```python
from build123d import *

# Parameters (mm, degrees)
SKETCH1_W           = 17.5
SKETCH1_H           = 22.5
BOSS_EXTRUDE1_DEPTH = 1.7
SKETCH2_W           = 6.644971707
SKETCH2_H           = 6.310332844
BOSS_EXTRUDE2_DEPTH = 2.75
SKETCH3_W           = 4.852263512
SKETCH3_H           = 6.382041172
BOSS_EXTRUDE3_DEPTH = 2


with BuildPart() as part:
    # Sketch1 → Boss-Extrude1 (new body)
    with BuildSketch(Plane(origin=(0, 0, 0), x_dir=(1, 0, 0), z_dir=(0, 1, 0))):
        with Locations((1.003989362, -11.25)):
            Rectangle(SKETCH1_W, SKETCH1_H)
    extrude(amount=BOSS_EXTRUDE1_DEPTH)

    # Sketch2 → Boss-Extrude2 (add)
    with BuildSketch(Plane(origin=(0, 1.7, 0), x_dir=(1, 0, 0), z_dir=(0, 1, 0))):
        with Locations((-2.473864536, -6.0870004)):
            Rectangle(SKETCH2_W, SKETCH2_H)
    extrude(amount=BOSS_EXTRUDE2_DEPTH)

    # Sketch3 → Boss-Extrude3 (add)
    with BuildSketch(Plane(origin=(0, 1.7, 0), x_dir=(1, 0, 0), z_dir=(0, 1, 0))):
        with Locations((1.577655984, -14.823465001)):
            Rectangle(SKETCH3_W, SKETCH3_H)
    extrude(amount=BOSS_EXTRUDE3_DEPTH)


solid = part.part
```
Geometry check sheet. Reference: the model listing, model coordinates, mm. A direction names the side the tool comes from. Give positions to 0.01 mm unless a question says otherwise; leave off trailing zeros. Loops run counter-clockwise (first coordinate to the right, second up) from the corner with the lowest first, then second, coordinate; pieces in that order, holes last. Notation, with made-up numbers: M 79.5,3.5 L 86.5,3.5 A16 ccw 86.5,22.5 Z; hole C 62.5,82.25 d6. An arc over 180 degrees is marked long. Write item = value, one per line. Start each with the question number.
1. Tool access check on faces 1 (the face through (2, 3, 18.014)), 2 (the face through (-0.848, 3, 15)), 3 (the face through (2, 3, 11.632)), 4 (the face through (4.004, 3, 15)), 5 (the face through (0.849, 3, 6)). Record the directions out of +Z, -Z, +X, -X, +Y, -Y that give a thin tool (end or side, any length) a straight path to the whole face; none if there is none.
2. Thickness scan on probe 1 along Y at (x, z) = (-1.5, 20.5); probe 2 along Y at (x, z) = (3.75, 12.25); probe 3 along Z at (x, y) = (-1.25, 2.35). Record the ranges inside material, lowest first.
3. Go/stop test with flat-tipped pins: P1, Ø1.5, axis at x = 5, z = 17, coming from the +Y side; P2, Ø5.5, axis at x = 2, z = 15, coming from the +Y side; P3, Ø1.4, axis at x = -3, y = 3, coming from the -Z side. Record where each tip stops, or that it passes through.
4. Section check D-D, the plane z = 21. Enter the section's corners in (x, y).
5. Section check C-C, the plane z = 5.25. Enter the section's corners in (x, y).
6. Section check B-B, the plane x = 2.75. Enter the section's corners in (y, z), plus the area to 3 significant figures.
7. Section check A-A, the plane y = 3.4. Enter the section's corners in (x, z), plus the area to 3 significant figures.
Values follow:
q1.face_1 = +Z, +X, -X, +Y
q1.face_2 = +Z, -X, +Y
q1.face_3 = +X, -X, +Y
q1.face_4 = +Z, -Z, +X, +Y
q1.face_5 = -Z, +X, +Y
q2.probe_1 = 0 to 1.7
q2.probe_2 = 0 to 3.7
q2.probe_3 = 2.93 to 9.24
q3.P1 = 1.7
q3.P2 = 3.7
q3.P3 = 2.93
q4.outline = M -7.75,0 L 9.75,0 L 9.75,1.7 L -7.75,1.7 Z
q5.outline = M -7.75,0 L 9.75,0 L 9.75,1.7 L 0.85,1.7 L 0.85,4.45 L -5.8,4.45 L -5.8,1.7 L -7.75,1.7 Z
q6.outline = M 0,0 L 1.7,0 L 1.7,11.63 L 3.7,11.63 L 3.7,18.01 L 1.7,18.01 L 1.7,22.5 L 0,22.5 Z
q6.area = 51.0 mm^2
q7.outline = M -5.8,2.93 L 0.85,2.93 L 0.85,9.24 L -5.8,9.24 Z; M -0.85,11.63 L 4,11.63 L 4,18.01 L -0.85,18.01 Z
q7.area = 72.9 mm^2
